from build123d import *

# Parameters (mm, degrees)
EXTRUDE_1_DEPTH     = 10
SKETCH_3_W          = 8
SKETCH_3_H          = 60
EXTRUDE_2_DEPTH     = 72
SKETCH_4_W          = 6
SKETCH_4_H          = 40
EXTRUDE_3_DEPTH     = 16
SKETCH_5_R          = 30
CUT_EXTRUDE_1_DEPTH = 77
SKETCH_6_R          = 2
CUT_EXTRUDE_2_DEPTH = 10
SKETCH_7_R          = 1.5
CUT_EXTRUDE_3_DEPTH = 10
SKETCH_8_W          = 8
SKETCH_8_H          = 16
EXTRUDE_4_DEPTH     = 60
CUT_EXTRUDE_4_DEPTH = 77


with BuildPart() as part:
    # 草图1 → 凸台-拉伸1 (new body)
    with BuildSketch(Plane(origin=(0, 0, 0), x_dir=(1, 0, 0), z_dir=(0, 1, 0))):
        with BuildLine():
            Line((-38, -75), (-38, 75))
            ThreePointArc((-38, 75), (0, 113), (38, 75))
            Line((38, 75), (38, -75))
            ThreePointArc((38, -75), (0, -113), (-38, -75))
        make_face()
    extrude(amount=EXTRUDE_1_DEPTH)

    # 草图3 → 凸台-拉伸2 (add)
    with BuildSketch(Plane(origin=(0, 10, 0), x_dir=(1, 0, 0), z_dir=(0, 1, 0))):
        with Locations((-34, -34)):
            Rectangle(SKETCH_3_W, SKETCH_3_H)
        with Locations((34, -34)):
            Rectangle(SKETCH_3_W, SKETCH_3_H)
    extrude(amount=EXTRUDE_2_DEPTH)

    # 草图4 → 凸台-拉伸3 (add)
    with BuildSketch(Plane(origin=(0, 10, 0), x_dir=(1, 0, 0), z_dir=(0, 1, 0))):
        with Locations((-35, 36)):
            Rectangle(SKETCH_4_W, SKETCH_4_H)
        with Locations((35, 36)):
            Rectangle(SKETCH_4_W, SKETCH_4_H)
    extrude(amount=EXTRUDE_3_DEPTH)

    # 草图5 → 切除-拉伸1 (cut, through all)
    with BuildSketch(Plane(origin=(38, 0, 0), x_dir=(0, 0, -1), z_dir=(1, 0, 0))):
        with Locations((-34, 97)):
            Circle(SKETCH_5_R)
    extrude(amount=-CUT_EXTRUDE_1_DEPTH, mode=Mode.SUBTRACT)

    # 草图6 → 切除-拉伸2 (cut)
    with BuildSketch(Plane.XY.offset(64)):
        with Locations((-34, 44)):
            Circle(SKETCH_6_R)
        with Locations((-34, 28)):
            Circle(SKETCH_6_R)
        with Locations((34, 44)):
            Circle(SKETCH_6_R)
        with Locations((34, 28)):
            Circle(SKETCH_6_R)
    extrude(amount=-CUT_EXTRUDE_2_DEPTH, mode=Mode.SUBTRACT)

    # 草图7 → 切除-拉伸3 (cut)
    with BuildSketch(Plane(origin=(0, 26, 0), x_dir=(1, 0, 0), z_dir=(0, 1, 0))):
        with Locations((-35, 26)):
            Circle(SKETCH_7_R)
        with Locations((-35, 46)):
            Circle(SKETCH_7_R)
        with Locations((35, 26)):
            Circle(SKETCH_7_R)
        with Locations((35, 46)):
            Circle(SKETCH_7_R)
    extrude(amount=-CUT_EXTRUDE_3_DEPTH, mode=Mode.SUBTRACT)

    # 草图8 → 凸台-拉伸4 (add)
    with BuildSketch(Plane(origin=(0, 10, 0), x_dir=(1, 0, 0), z_dir=(0, 1, 0))):
        with Locations((-34, 64)):
            Rectangle(SKETCH_8_W, SKETCH_8_H)
        with Locations((34, 64)):
            Rectangle(SKETCH_8_W, SKETCH_8_H)
    extrude(amount=EXTRUDE_4_DEPTH)

    # 草图9 → 切除-拉伸4 (cut, through all)
    with BuildSketch(Plane(origin=(38, 0, 0), x_dir=(0, 0, -1), z_dir=(1, 0, 0))):
        with BuildLine():
            Line((56, 62), (56, 75))
            Line((56, 75), (72, 75))
            Line((72, 75), (72, 62))
            ThreePointArc((72, 62), (64, 70), (56, 62))
        make_face()
    extrude(amount=-CUT_EXTRUDE_4_DEPTH, mode=Mode.SUBTRACT)


solid = part.part
Geometry check sheet. Reference: the model listing, model coordinates, mm. A direction names the side the tool comes from. Coordinates: 2 decimals unless noted, no trailing zeros. Order: outer loops, then holes, each group sorted by start corner. A loop starts at its lowest first (then second) coordinate and runs counter-clockwise, first axis right, second up. Notation, with made-up numbers: (51, 22.5) - (56, 22.5) arc R17 cw to (56, 27.5) - close; hole circle Ø2 at (88, -5). An arc over 180 degrees is marked (long way). Answer in a Markdown table with one row per item. Add a question column.
1) Release check for a two-part mould opening along Y. For faces 1 (the flat face through (1, 0, -2)), 2 (the flat face through (34, 28, 54)), 3 (the flat face through (-34, 36, -72)), 4 (the flat face through (35, 26, -36)) record: +Y half, -Y half, draft (parallel to the pull), parting line (faces both ways), or undercut.
2) Gauge pin test, flat ends, axial feed: P1, Ø3, axis at x = -35.5, y = 17, coming from the +Z side; P2, Ø9, axis at x = -33, y = 44.5, coming from the -Z side; P3, Ø2.5, axis at x = 35, z = -26, coming from the +Y side. Record the tip position at first contact, or that the pin passes through.
3) Cross-section at B-B, the plane x = 0. Record the cut outline in (y, z), then the cut area to 3 significant figures.
4) Cross-section at C-C, the plane z = 48.5. Record the cut outline in (x, y).
5) Cross-section at A-A, the plane z = -52.5. Record the cut outline in (x, y).
6) Material ranges on line 1 along X through (y, z) = (23, -46); line 2 along Z through (x, y) = (35, 23); line 3 along Y through (x, z) = (-34, 62.25), recorded low to high. Write a range as [from, to].
7) Set-up check for faces 5 (the flat face through (-30, 40, -64)), 6 (the cylindrical face through (34.923, 42.226, 59.07)), 7 (the flat face through (34, 36, -72)), 8 (the flat face through (-35, 26, -36)): record each of +Z, -Z, +X, -X, +Y, -Y from which the full face is reachable in a straight line by a thin tool's end or side.
8) Cross-section at D-D, the plane x = 27.5. Record the cut outline in (y, z).
Check result:
| question | item | result |
|---|---|---|
| 1 | face 1 | -Y half |
| 1 | face 2 | undercut |
| 1 | face 3 | draft |
| 1 | face 4 | +Y half |
| 2 | P1 | stops at z = 64 |
| 2 | P2 | stops at z = -72 |
| 2 | P3 | stops at y = 16 |
| 3 | outline | (0, -113) - (10, -113) - (10, 113) - (0, 113) - close |
| 3 | area | 2,260 mm² |
| 4 | outline | (-38, 0) - (38, 0) - (38, 70.74) - (30, 70.74) - (30, 10) - (-30, 10) - (-30, 70.74) - (-38, 70.74) - close |
| 5 | outline | (-38, 0) - (38, 0) - (38, 26) - (32, 26) - (32, 10) - (-32, 10) - (-32, 26) - (-38, 26) - close |
| 6 | line 1 | x = [-38, -36.5], [-33.5, -32], [32, 33.5], [36.5, 38] |
| 6 | line 2 | z = [-72, -47.5], [-44.5, -27.5], [-24.5, -16], [4, 64] |
| 6 | line 3 | y = [0, 26], [30, 42], [46, 82] |
| 7 | face 5 | +Z, -Z, +Y |
| 7 | face 6 | +Z |
| 7 | face 7 | -Z, +X, -X, +Y |
| 7 | face 8 | +X, -X, +Y |
| 8 | outline | (0, -101.22) - (10, -101.22) - (10, 101.22) - (0, 101.22) - close |
